Check sheet for the drawn part. Datum: minimum x, y, z corner. Units: mm. A direction names the side the tool comes from. Give positions to 0.01 mm unless a question says otherwise; leave off trailing zeros. Write each loop counter-clockwise with the first axis right and the second up, starting at its lowest first coordinate (ties: lowest second). Pieces come first, ordered by that corner, then holes. Notation, with made-up numbers: (-21, 26.25) -> (36, 26.25) arc R20 ccw to (36, 40.25) -> close; hole circle Ø2 at (0.5, -9.5). An arc over 180 degrees is marked (long way). Write item = value, one per line. Start each with the question number.
1. Cross-section at A-A, the plane x = 22.45. Record the cut outline in (y, z).
2. Mould release check, pull along X, two halves, no side actions. Record for the marked faces 1, 2, 3 and 4: pulls with the +X half, pulls with the -X half, needs draft (parallel to the pull), parting line crosses it, or undercut.
3. Cross-section at D-D, the plane y = 15.5. Record the cut outline in (x, z).
4. Thickness scan on line 1 along X through (y, z) = (7.5, 7.75); line 2 along Z through (x, y) = (22.5, 31.5); line 3 along Y through (x, z) = (23, 11.75). Record the ranges inside material, lowest first.
5. Cross-section at B-B, the plane y = 44. Record the cut outline in (x, z).
6. Set-up check for the marked faces 5, 6 and 7: record each of +Z, -Z, +X, -X, +Y, -Y from which the full face is reachable in a straight line by a thin tool's end or side.
7. Depth check by flat-ended pin: P1, Ø1.5, axis at x = 11.5, z = 12.5, coming from the +Y side; P2, Ø5, axis at x = 2, z = 10.5, coming from the -Y side; P3, Ø5, axis at y = 22, z = 6.5, coming from the -X side. Enter the tip coordinate at first touch or a pass-through.
8. Cross-section at C-C, the plane z = 6.25. Record the cut outline in (x, y), plus the area to 3 significant figures.
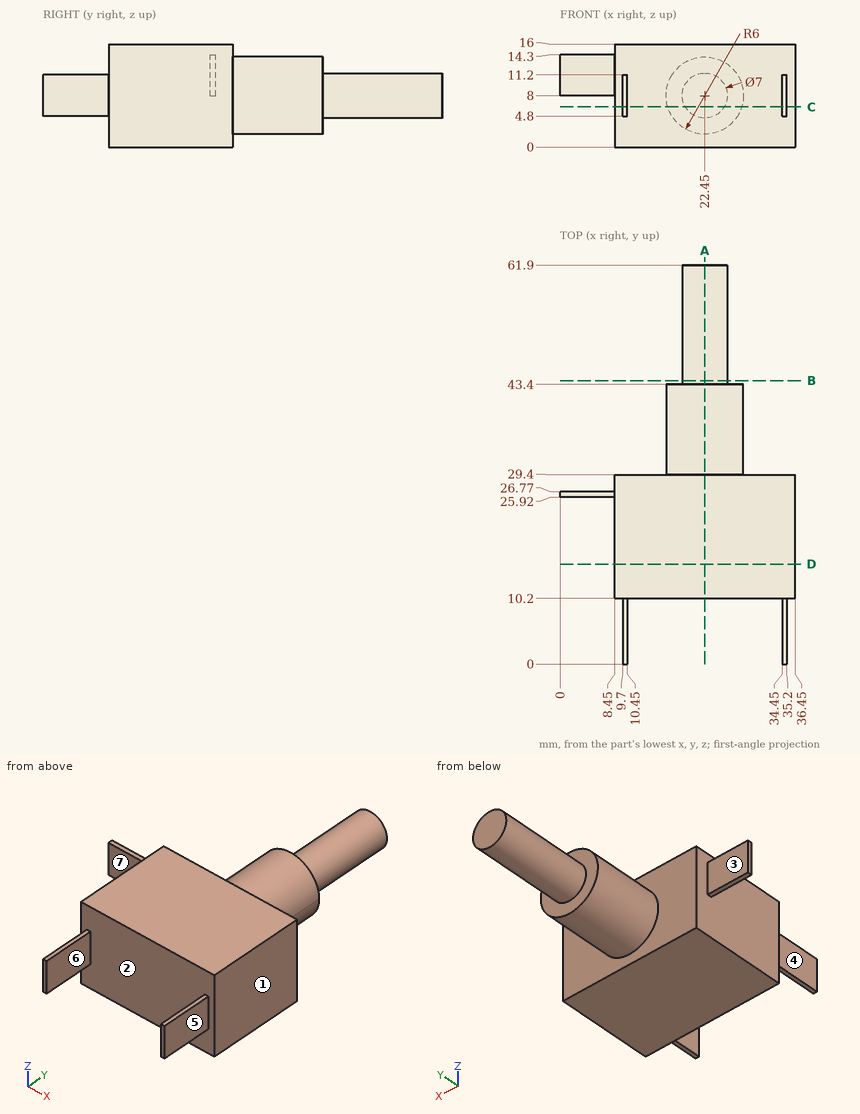
Answers:
q1.outline = (10.2, 0) -> (29.4, 0) -> (29.4, 2) -> (43.4, 2) -> (43.4, 4.5) -> (61.9, 4.5) -> (61.9, 11.5) -> (43.4, 11.5) -> (43.4, 14) -> (29.4, 14) -> (29.4, 16) -> (10.2, 16) -> close
q2.face_1 = pulls with the +X half
q2.face_2 = undercut
q2.face_3 = needs draft
q2.face_4 = pulls with the -X half
q3.outline = (8.45, 0) -> (36.45, 0) -> (36.45, 16) -> (8.45, 16) -> close
q4.line_1 = 9.7 to 10.45, 34.45 to 35.2
q4.line_2 = 2 to 14
q4.line_3 = 10.2 to 43.4
q5.outline = circle Ø7 at (22.45, 8)
q6.face_5 = +Z, -Z, +X, -Y
q6.face_6 = +Z, -Z, -Y
q6.face_7 = +Z, -Z, -X, -Y
q7.P1 = 29.4
q7.P2 = 25.92
q7.P3 = 8.45
q8.outline = (8.45, 10.2) -> (9.7, 10.2) -> (9.7, 0) -> (10.45, 0) -> (10.45, 10.2) -> (34.45, 10.2) -> (34.45, 0) -> (35.2, 0) -> (35.2, 10.2) -> (36.45, 10.2) -> (36.45, 29.4) -> (28.19, 29.4) -> (28.19, 43.4) -> (25.48, 43.4) -> (25.48, 61.9) -> (19.42, 61.9) -> (19.42, 43.4) -> (16.71, 43.4) -> (16.71, 29.4) -> (8.45, 29.4) -> close
q8.area = 826 mm^2
